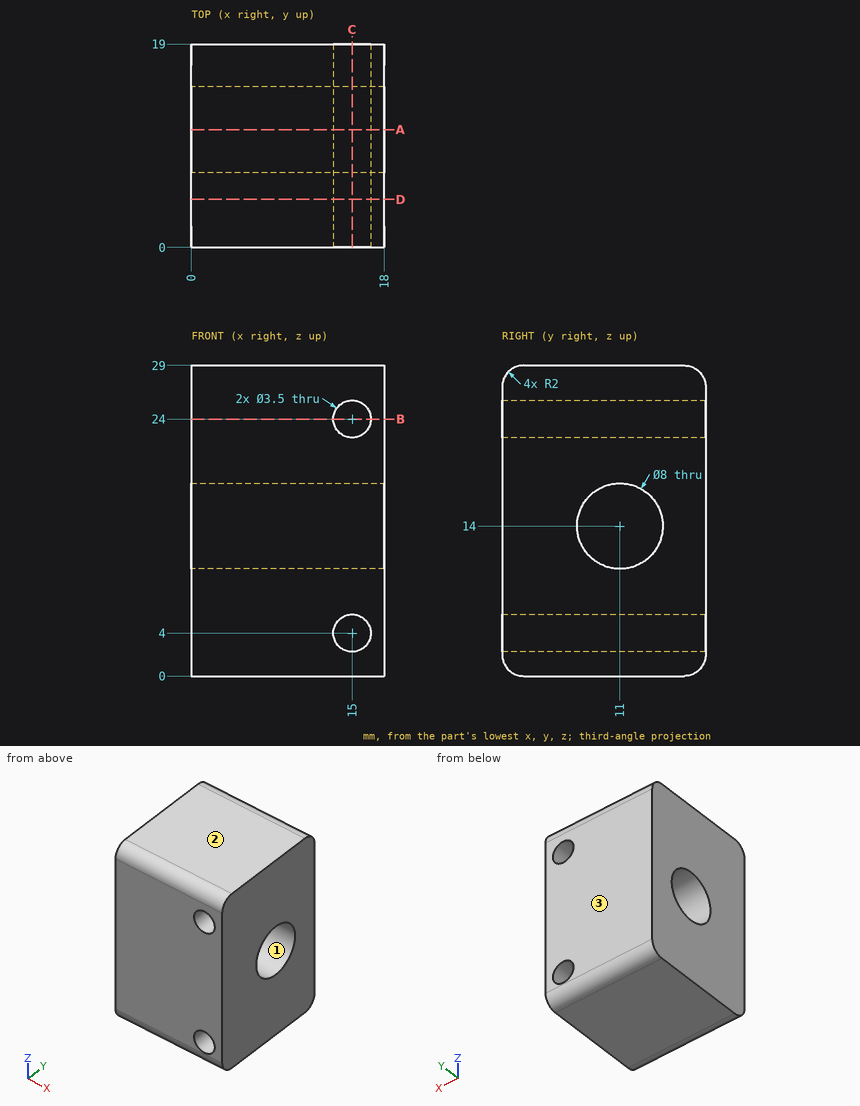
Source: three-view drawing plus pictorial views. Frame: mm from the lowest corner of the part. Round coordinates to 2 decimals unless told otherwise and drop trailing zeros. Loops run counter-clockwise (first coordinate to the right, second up) from the corner with the lowest first, then second, coordinate; pieces in that order, holes last.
1. Ray query, L1, parallel to X at y = 14, z = 4; L2, parallel to Z at x = 15.5, y = 5.5; L3, parallel to Z at x = 16.25, y = 8.5. Return the intervals inside material, ascending.
2. Section query B-B on z = 24. Output: boundary loops of the cut face in (x, y).
3. Section query A-A on y = 11. Output: boundary loops of the cut face in (x, z).
4. Mould query, pull axis Z, two halves, no side actions, for the marked faces 1, 2 and 3. Classes: released by +Z, released by -Z, zero draft, split by the parting line, or undercut.
5. Section query C-C on x = 15. Output: boundary loops of the cut face in (y, z), and give its area (3 significant figures).
6. Section query D-D on y = 4.5. Output: boundary loops of the cut face in (x, z), and give its area (3 significant figures).
Answers below:
1. L1: x = 0 to 13.25, 16.75 to 18
1. L2: z = 0 to 2.32, 5.68 to 22.32, 25.68 to 29
1. L3: z = 0 to 2.78, 5.22 to 10.88, 17.12 to 22.78, 25.22 to 29
2. outline: (0, 0) - (13.25, 0) - (13.25, 19) - (0, 19) - close; (16.75, 0) - (18, 0) - (18, 19) - (16.75, 19) - close
3. outline: (0, 0) - (18, 0) - (18, 10) - (0, 10) - close; (0, 18) - (18, 18) - (18, 29) - (0, 29) - close; hole circle Ø3.5 at (15, 4); hole circle Ø3.5 at (15, 24)
4. face 1: undercut
4. face 2: released by +Z
4. face 3: zero draft
5. outline: (0, 2) arc R2 ccw to (2, 0) - (17, 0) arc R2 ccw to (19, 2) - (19, 2.25) - (0, 2.25) - close; (0, 5.75) - (19, 5.75) - (19, 22.25) - (0, 22.25) - close; (0, 25.75) - (19, 25.75) - (19, 27) arc R2 ccw to (17, 29) - (2, 29) arc R2 ccw to (0, 27) - close; hole circle Ø8 at (11, 14)
5. area: 364 mm2
6. outline: (0, 0) - (18, 0) - (18, 29) - (0, 29) - close; hole circle Ø3.5 at (15, 4); hole circle Ø3.5 at (15, 24)
6. area: 503 mm2
